```python
from build123d import *

# Parameters (mm, degrees)
F0_W     = 114.3
F0_H     = 88.9
F1_DEPTH = 25.4
F3_DEPTH = 25.4
F5_DEPTH = 50.8


with BuildPart() as f1:
    # F0 (on Front) → F1 (new body)
    with BuildSketch(Plane.XZ):
        with Locations((-0.7014218356, -5.7260454797)):
            Rectangle(F0_W, F0_H)
    extrude(amount=F1_DEPTH)

    # F2 (on face) → F3 (join)
    with BuildSketch(Plane.XZ.offset(25.4)):
        Polygon((-19.7514218356, 38.7239545203), (-57.8514218356, 38.7239545203), (-57.8514218356, -50.1760454797), (56.4485781644, -50.1760454797), align=None)
    extrude(amount=F3_DEPTH)

    # F4 (on face) → F5 (cut)
    with BuildSketch(Plane.XZ.offset(50.8)):
        with BuildLine():
            ThreePointArc((-8.8132691571, 25.9627763954), (-25.6243984679, 17.9503661228), (-32.4514218356, 0.6239545203))
            Line((-32.4514218356, 0.6239545203), (-7.0514218356, 0.6239545203))
            Line((-7.0514218356, 0.6239545203), (-7.0514218356, 23.9072878537))
            Line((-7.0514218356, 23.9072878537), (-8.8132691571, 25.9627763954))
        make_face()
        with BuildLine():
            ThreePointArc((-32.4514218356, 0.6239545203), (-25.0119340777, -17.3365577218), (-7.0514218356, -24.7760454797))
            Line((-7.0514218356, -24.7760454797), (-7.0514218356, 0.6239545203))
            Line((-7.0514218356, 0.6239545203), (-32.4514218356, 0.6239545203))
        make_face()
        with BuildLine():
            Line((-7.0514218356, 0.6239545203), (-7.0514218356, -24.7760454797))
            ThreePointArc((-7.0514218356, -24.7760454797), (8.7994722887, -19.2231902481), (17.7198372506, -4.9925144135))
            Line((17.7198372506, -4.9925144135), (-7.0514218356, 23.9072878537))
            Line((-7.0514218356, 23.9072878537), (-7.0514218356, 0.6239545203))
        make_face()
        with BuildLine():
            Line((-7.0514218356, 23.9072878537), (17.7198372506, -4.9925144135))
            ThreePointArc((17.7198372506, -4.9925144135), (18.1909035405, -2.2018214095), (18.3485781644, 0.6239545203))
            ThreePointArc((18.3485781644, 0.6239545203), (10.2749897668, 19.1969311526), (-8.8132691571, 25.9627763954))
            Line((-8.8132691571, 25.9627763954), (-7.0514218356, 23.9072878537))
        make_face()
    extrude(amount=-F5_DEPTH, mode=Mode.SUBTRACT)


solid = f1.part
```
Work out the finished part from the listing and answer in its coordinate system (mm). A direction names the side the tool comes from. Give positions to 0.01 mm unless a question says otherwise; leave off trailing zeros. Order: outer loops, then holes, each group sorted by start corner. A loop starts at its lowest first (then second) coordinate and runs counter-clockwise, first axis right, second up.
1. Straight lines are drawn through the part: L1, parallel to X at y = -8, z = 0.5; L2, parallel to Y at x = 28.5, z = -11; L3, parallel to Z at x = 9, y = -22.5. For each, find the intervals that lie inside material, in ascending order.
Result sheet:
L1: x = -57.85 to -32.45, 18.35 to 56.45
L2: y = -25.4 to 0
L3: z = -50.18 to -19.06, 20.31 to 38.72
2. Section B-B, the plane x = -15 is taken. Determine the outline of the cut face in (y, z).
Result sheet:
outline: (-50.8, -50.18) - (0, -50.18) - (0, -23.5) - (-50.8, -23.5) - close; (-50.8, 24.75) - (0, 24.75) - (0, 38.72) - (-25.4, 38.72) - (-25.4, 33.18) - (-50.8, 33.18) - close
3. For faces 1 (the flat face through (37.355, -37.922, -27.901)), 2 (the flat face through (-14, -50.8, -25)), determine the directions among +Z, -Z, +X, -X, +Y, -Y from which every point of the face is accessible in a straight line to the end or side of a thin tool.
Result sheet:
face 1: +Z, +X, -Y
face 2: +Z, -Z, +X, -X, -Y
4. Section C-C, the plane y = -8.5 is taken. Determine the outline of the cut face in (x, z), and give its area (3 significant figures).
Result sheet:
outline: (-57.85, -50.18) - (56.45, -50.18) - (56.45, 38.72) - (-57.85, 38.72) - close; hole circle Ø50.8 at (-7.05, 0.62)
area: 8,130 mm2
5. Section D-D, the plane y = -27 is taken. Determine the outline of the cut face in (x, z), and give its area (3 significant figures).
Result sheet:
outline: (-57.85, -50.18) - (56.45, -50.18) - (17.72, -4.99) arc R25.4 cw (long way) to (-8.81, 25.96) - (-19.75, 38.72) - (-57.85, 38.72) - close
area: 5,040 mm2
6. Section A-A, the plane z = 16 is taken. Determine the outline of the cut face in (x, y).
Result sheet:
outline: (-57.85, -50.8) - (-27.27, -50.8) - (-27.27, 0) - (-57.85, 0) - close; (13.17, -25.4) - (56.45, -25.4) - (56.45, 0) - (13.17, 0) - close
7. The mould has two halves that part along Z. Classify faces 3 (the flat face through (-2, -25, -50.176)), 4 (the flat face through (35, -25.4, 15)), 5 (the flat face through (-14.206, -37.922, 32.254)): released by +Z, released by -Z, zero draft, split by the parting line, or undercut.
Result sheet:
face 3: released by -Z
face 4: zero draft
face 5: released by +Z
8. This flat-tipped pin is pushed along its axis until it touches: P1, Ø8, axis at x = 34.5, z = 7, coming from the -Y side. Where does it stop, or does it pass through?
Result sheet:
P1: stops at y = -25.4
